Geometry: see drawing. Coordinates: mm, zero at the bounding-box minimum. A direction names the side the tool comes from. Coordinates: 2 decimals unless noted, no trailing zeros. Loops run counter-clockwise (first coordinate to the right, second up) from the corner with the lowest first, then second, coordinate; pieces in that order, holes last. Notation, with made-up numbers: (66, 30.25) - (93, 30.25) arc R10 ccw to (93, 48.25) - close; hole circle Ø6 at (-32.5, 23.5). An arc over 180 degrees is marked (long way). Answer in a Markdown table with one row per item.
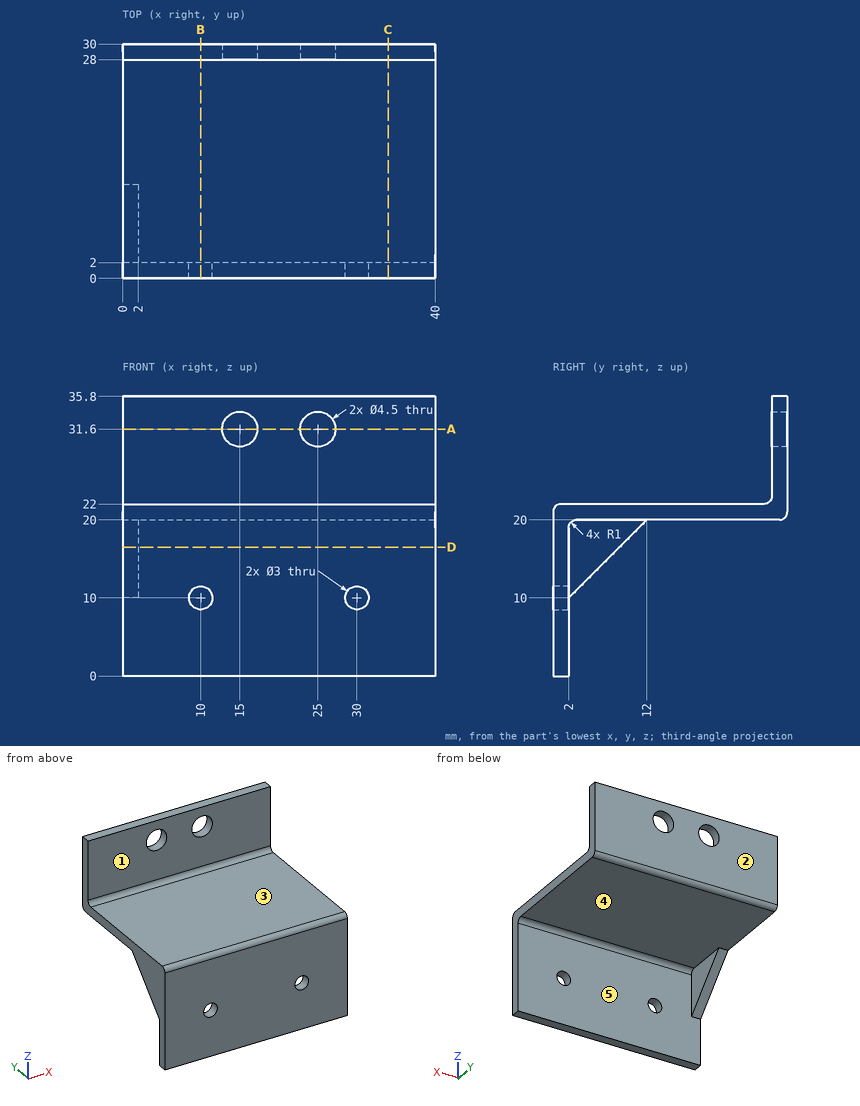
(1) Cut plane C-C on x = 34. Output: boundary loops of the cut face in (y, z).
Verdict:
| item | result |
|---|---|
| outline | (0, 0) - (2, 0) - (2, 19) arc R1 cw to (3, 20) - (29, 20) arc R1 ccw to (30, 21) - (30, 35.8) - (28, 35.8) - (28, 23) arc R1 cw to (27, 22) - (1, 22) arc R1 ccw to (0, 21) - close |
(2) Ray query, probe 1 along X at (y, z) = (29, 31.6); probe 2 along X at (y, z) = (1.65, 10); probe 3 along Z at (x, y) = (12.5, 23.25). Return the intervals inside material, ascending.
Verdict:
| item | result |
|---|---|
| probe 1 | x = 0 to 12.75, 17.25 to 22.75, 27.25 to 40 |
| probe 2 | x = 0 to 8.5, 11.5 to 28.5, 31.5 to 40 |
| probe 3 | z = 20 to 22 |
(3) Cut plane B-B on x = 10. Output: boundary loops of the cut face in (y, z).
Verdict:
| item | result |
|---|---|
| outline | (0, 0) - (2, 0) - (2, 8.5) - (0, 8.5) - close; (0, 11.5) - (2, 11.5) - (2, 19) arc R1 cw to (3, 20) - (29, 20) arc R1 ccw to (30, 21) - (30, 35.8) - (28, 35.8) - (28, 23) arc R1 cw to (27, 22) - (1, 22) arc R1 ccw to (0, 21) - close |
(4) Cut plane D-D on z = 16.5. Output: boundary loops of the cut face in (x, y), then the cut area to 3 significant figures.
Verdict:
| item | result |
|---|---|
| outline | (0, 0) - (40, 0) - (40, 2) - (2, 2) - (2, 8.5) - (0, 8.5) - close |
| area | 93.0 mm² |
(5) Pull-direction query (Z, two-part tool) for the marked faces 3, 4 and 5; classes: pulls with the +Z half, pulls with the -Z half, needs draft (parallel to the pull), parting line crosses it, or undercut.
Verdict:
| item | result |
|---|---|
| face 3 | pulls with the +Z half |
| face 4 | pulls with the -Z half |
| face 5 | needs draft |
(6) Cut plane A-A on z = 31.6. Output: boundary loops of the cut face in (x, y), then the cut area to 3 significant figures.
Verdict:
| item | result |
|---|---|
| outline | (0, 28) - (12.75, 28) - (12.75, 30) - (0, 30) - close; (17.25, 28) - (22.75, 28) - (22.75, 30) - (17.25, 30) - close; (27.25, 28) - (40, 28) - (40, 30) - (27.25, 30) - close |
| area | 62.0 mm² |
(7) First-contact query: pin 1 Ø10 at (x, y) = (17.5, 15.5) entering from +Z; pin 2 Ø9.5 at (x, z) = (15, 12.5) entering from +Y; pin 3 Ø4 at (x, y) = (13, 21) entering from -Z. Flat tips, straight axial feed; report the tip coordinate or a pass-through.
Verdict:
| item | result |
|---|---|
| pin 1 | stops at z = 22 |
| pin 2 | stops at y = 2 |
| pin 3 | stops at z = 20 |
(8) Access query for the marked faces 1 and 2. Directions: +Z, -Z, +X, -X, +Y, -Y. A direction counts if a zero-diameter tool reaches every point of the face in a straight line with its end or side. Return the directions, or none.
Verdict:
| item | result |
|---|---|
| face 1 | +Z, +X, -X, -Y |
| face 2 | +Z, -Z, +X, -X, +Y |
